The model under review builds one solid part; all positions refer to its coordinate system, in mm. A direction names the side the tool comes from. Coordinates: 2 decimals unless noted, no trailing zeros. Order: outer loops, then holes, each group sorted by start corner. A loop starts at its lowest first (then second) coordinate and runs counter-clockwise, first axis right, second up. Notation, with made-up numbers: (53.5, -6) -> (105.5, -6) arc R15 cw to (105.5, 22) -> close; hole circle Ø5 at (23, 19). An arc over 180 degrees is marked (long way). Use one line per item in the form item = value.
from build123d import *

# Parameters (mm, degrees)
F0_R     = 29.412961
F1_DEPTH = 12.7
F0_R_2   = 22.225
F2_DEPTH = 63.5
F0_R_3   = 6.35
F3_DEPTH = 66.675
F4_DEPTH = 92.075
F5_DEPTH = 25.4


with BuildPart() as f1:
    # F0 (on Top) → F1 (new body)
    with BuildSketch(Plane.XY):
        with BuildLine():
            Line((-23.65, -30), (23.65, -30))
            ThreePointArc((23.65, -30), (28.140128, -28.140128), (30, -23.65))
            Line((30, -23.65), (30, 23.65))
            ThreePointArc((30, 23.65), (28.140128, 28.140128), (23.65, 30))
            Line((23.65, 30), (-23.65, 30))
            ThreePointArc((-23.65, 30), (-28.140128, 28.140128), (-30, 23.65))
            Line((-30, 23.65), (-30, -23.65))
            ThreePointArc((-30, -23.65), (-28.140128, -28.140128), (-23.65, -30))
        make_face()
        Circle(F0_R, mode=Mode.SUBTRACT)
    extrude(amount=F1_DEPTH)

    # F0 (on Top) → F2 (join)
    with BuildSketch(Plane.XY):
        Circle(F0_R)
        Circle(F0_R_2, mode=Mode.SUBTRACT)
    extrude(amount=F2_DEPTH)

    # F0 (on Top) → F3 (join)
    with BuildSketch(Plane.XY):
        Circle(F0_R_2)
        Circle(F0_R_3, mode=Mode.SUBTRACT)
    extrude(amount=F3_DEPTH)

    # F0 (on Top) → F4 (join)
    with BuildSketch(Plane.XY):
        Circle(F0_R_3)
    extrude(amount=F4_DEPTH)

    # F0 (on Top) → F5 (cut)
    with BuildSketch(Plane.XY):
        Circle(F0_R_3)
    extrude(amount=F5_DEPTH, mode=Mode.SUBTRACT)


solid = f1.part
Item 1: Clearance check with flat-ended pins moving along their axes: pin 1 (6 mm diameter, centred on x = 2.5, z = 16, fed in from -Y); pin 2 (3 mm diameter, centred on x = 10, y = -20.5, fed in from +Z) (3 decimals); pin 3 (1 mm diameter, centred on y = -8, z = 41.5, fed in from -X). State where each tip first meets the part, or that it passes through.
Results found:
pin_1 = -29.41
pin_2 = 66.675
pin_3 = -28.44
Item 2: To check wall thickness, follow L1, parallel to Y at x = 0, z = 10.75; L2, parallel to Y at x = 0, z = 20; L3, parallel to Z at x = -14.5, y = -26.5. State the ranges of each line that lie inside material, in increasing order. Write a range as from..to.
Results found:
L1 = -30..-6.35, 6.35..30
L2 = -29.41..-6.35, 6.35..29.41
L3 = 0..12.7
Item 3: We need section A-A (z = 11). Write out the cut boundary in (x, y).
Results found:
outline = (-30, -23.65) arc R6.35 ccw to (-23.65, -30) -> (23.65, -30) arc R6.35 ccw to (30, -23.65) -> (30, 23.65) arc R6.35 ccw to (23.65, 30) -> (-23.65, 30) arc R6.35 ccw to (-30, 23.65) -> close; hole circle Ø12.7 at (0, 0)
Item 4: Tool access review of faces 5 (the face through (0, 30, 6)), 6 (the face through (5, -5, 66.675)): name each direction out of +Z, -Z, +X, -X, +Y, -Y from which nothing blocks a thin tool from reaching the whole face with its end or side.
Results found:
face_5 = +Z, -Z, +X, -X, +Y
face_6 = +Z
Item 5: We need section B-B (y = 0). Write out the cut boundary in (x, z) (3 decimals).
Results found:
outline = (-30, 0) -> (-6.35, 0) -> (-6.35, 25.4) -> (6.35, 25.4) -> (6.35, 0) -> (30, 0) -> (30, 12.7) -> (29.413, 12.7) -> (29.413, 63.5) -> (22.225, 63.5) -> (22.225, 66.675) -> (6.35, 66.675) -> (6.35, 92.075) -> (-6.35, 92.075) -> (-6.35, 66.675) -> (-22.225, 66.675) -> (-22.225, 63.5) -> (-29.413, 63.5) -> (-29.413, 12.7) -> (-30, 12.7) -> close
Item 6: Draft analysis for pull direction X (two halves, no side actions). For faces 1 (the face through (-1.38, -6.2, 12.52)), 2 (the face through (-6.376, -28.714, 37.744)), 3 (the face through (0, 0, 25.4)), 4 (the face through (0, 0, 92.075)), state which applies: released by +X, released by -X, zero draft, split by the parting line, or undercut.
Results found:
face_1 = undercut
face_2 = split by the parting line
face_3 = undercut
face_4 = zero draft
Item 7: We need section D-D (z = 85). Write out the cut boundary in (x, y).
Results found:
outline = circle Ø12.7 at (0, 0)
